Could you check a few things on this model? Use its own coordinates, in mm. Give positions to 0.01 mm unless a question says otherwise; leave off trailing zeros. Order: outer loops, then holes, each group sorted by start corner. A loop starts at its lowest first (then second) coordinate and runs counter-clockwise, first axis right, second up.
(1) Imagine slicing it at A-A, the plane z = 534. Write out the boundary of the cut face in (x, y).
(2) Imagine slicing it at B-B, the plane z = 510. Write out the boundary of the cut face in (x, y), then the cut area to 3 significant figures.
(3) If I drill on probe 1 along X at (y, z) = (39.1, 534); probe 2 along Z at (x, y) = (-13, 35.1); probe 3 along Z at (x, y) = (-14.5, 36.75), over which ranges is the centre line in solid material (lowest first)?
(4) Will these pins go through, and if not, where does the flat tip stop? pin 1 (1.5 mm diameter, centred on y = 37.5, z = 487.5, fed in from -X); pin 2 (3 mm diameter, centred on y = 39.5, z = 473, fed in from +X); pin 3 (3.5 mm diameter, centred on x = 12.39, z = 491.65, fed in from +Y); pin 4 (2.5 mm diameter, centred on x = -7.63, z = 499.9, fed in from -Y).
(5) Imagine slicing it at C-C, the plane y = 39.5. State how many separate pieces and enclosed holes the cut face has, then the cut area to 3 significant figures.
from build123d import *

# Parameters (mm, degrees)
PLACA_START                 = 34.5
SK_PLACA_W                  = 50
SK_PLACA_H                  = 36
PLACA_DEPTH                 = 6
EXTREMO_START               = 34.5
SK_EXTREMO_R                = 25
EXTREMO_DEPTH               = 6
PASANTES_M2_5_CUBO_J5_START = 34.5
SK_PASANTES_M2_5_CUBO_J5_R  = 1.45
PASANTES_M2_5_CUBO_J5_DEPTH = 6
CAJAS_M2_5_J5_START         = 38
SK_CAJAS_M2_5_J5_R          = 2.75
CAJAS_M2_5_J5_DEPTH         = 2.5
EXTENSION_PESTANAS_START    = 34.5
SK_EXTENSION_PESTANAS_W     = 50
SK_EXTENSION_PESTANAS_H     = 19
EXTENSION_PESTANAS_DEPTH    = 6
PASANTES_M4_REPISA_START    = 34.5
SK_PASANTES_M4_REPISA_R     = 2.25
PASANTES_M4_REPISA_DEPTH    = 6
PASANTE_M3_CINCHO_START     = 34.5
SK_PASANTE_M3_CINCHO_R      = 1.7
PASANTE_M3_CINCHO_DEPTH     = 6


with BuildPart() as part:
    # Sk_Placa → Placa (new body)
    with BuildSketch(Plane(origin=(0, 0, 0), x_dir=(1, 0, 0), z_dir=(0, 1, 0)).offset(PLACA_START)):
        with Locations((0, -508)):
            Rectangle(SK_PLACA_W, SK_PLACA_H)
    extrude(amount=PLACA_DEPTH)

    # Sk_Extremo → Extremo (add)
    with BuildSketch(Plane(origin=(0, 0, 0), x_dir=(1, 0, 0), z_dir=(0, 1, 0)).offset(EXTREMO_START)):
        with Locations((0, -490)):
            Circle(SK_EXTREMO_R)
    extrude(amount=EXTREMO_DEPTH)

    # Sk_Pasantes_M2-5_cubo_J5 → Pasantes_M2-5_cubo_J5 (cut)
    with BuildSketch(Plane(origin=(0, 0, 0), x_dir=(1, 0, 0), z_dir=(0, 1, 0)).offset(PASANTES_M2_5_CUBO_J5_START)):
        with Locations(Location((12.390194253, -491.653204878, 0), (0, 0, 270))):
            Circle(SK_PASANTES_M2_5_CUBO_J5_R)
        with Locations(Location((4.763379704, -501.55682542, 0), (0, 0, 270))):
            Circle(SK_PASANTES_M2_5_CUBO_J5_R)
        with Locations(Location((-7.626814549, -499.903620542, 0), (0, 0, 270))):
            Circle(SK_PASANTES_M2_5_CUBO_J5_R)
        with Locations(Location((-12.390194253, -488.346795122, 0), (0, 0, 270))):
            Circle(SK_PASANTES_M2_5_CUBO_J5_R)
        with Locations(Location((-4.763379704, -478.44317458, 0), (0, 0, 270))):
            Circle(SK_PASANTES_M2_5_CUBO_J5_R)
        with Locations(Location((7.626814549, -480.096379458, 0), (0, 0, 270))):
            Circle(SK_PASANTES_M2_5_CUBO_J5_R)
    extrude(amount=PASANTES_M2_5_CUBO_J5_DEPTH, mode=Mode.SUBTRACT)

    # Sk_Cajas_M2-5_J5 → Cajas_M2-5_J5 (cut)
    with BuildSketch(Plane(origin=(0, 0, 0), x_dir=(1, 0, 0), z_dir=(0, 1, 0)).offset(CAJAS_M2_5_J5_START)):
        with Locations(Location((12.390194253, -491.653204878, 0), (0, 0, 270))):
            Circle(SK_CAJAS_M2_5_J5_R)
        with Locations(Location((4.763379704, -501.55682542, 0), (0, 0, 270))):
            Circle(SK_CAJAS_M2_5_J5_R)
        with Locations(Location((-7.626814549, -499.903620542, 0), (0, 0, 270))):
            Circle(SK_CAJAS_M2_5_J5_R)
        with Locations(Location((-12.390194253, -488.346795122, 0), (0, 0, 270))):
            Circle(SK_CAJAS_M2_5_J5_R)
        with Locations(Location((-4.763379704, -478.44317458, 0), (0, 0, 270))):
            Circle(SK_CAJAS_M2_5_J5_R)
        with Locations(Location((7.626814549, -480.096379458, 0), (0, 0, 270))):
            Circle(SK_CAJAS_M2_5_J5_R)
    extrude(amount=CAJAS_M2_5_J5_DEPTH, mode=Mode.SUBTRACT)

    # Sk_Extension_pestanas → Extension_pestanas (add)
    with BuildSketch(Plane(origin=(0, 0, 0), x_dir=(1, 0, 0), z_dir=(0, 1, 0)).offset(EXTENSION_PESTANAS_START)):
        with Locations((0, -535.5)):
            Rectangle(SK_EXTENSION_PESTANAS_W, SK_EXTENSION_PESTANAS_H)
    extrude(amount=EXTENSION_PESTANAS_DEPTH)

    # Sk_Pasantes_M4_repisa → Pasantes_M4_repisa (cut)
    with BuildSketch(Plane(origin=(0, 0, 0), x_dir=(1, 0, 0), z_dir=(0, 1, 0)).offset(PASANTES_M4_REPISA_START)):
        with Locations(Location((-15, -534, 0), (0, 0, 270))):
            Circle(SK_PASANTES_M4_REPISA_R)
        with Locations(Location((15, -534, 0), (0, 0, 270))):
            Circle(SK_PASANTES_M4_REPISA_R)
    extrude(amount=PASANTES_M4_REPISA_DEPTH, mode=Mode.SUBTRACT)

    # Sk_Pasante_M3_cincho → Pasante_M3_cincho (cut)
    with BuildSketch(Plane(origin=(0, 0, 0), x_dir=(1, 0, 0), z_dir=(0, 1, 0)).offset(PASANTE_M3_CINCHO_START)):
        with Locations(Location((-15, -510, 0), (0, 0, 270))):
            Circle(SK_PASANTE_M3_CINCHO_R)
    extrude(amount=PASANTE_M3_CINCHO_DEPTH, mode=Mode.SUBTRACT)


solid = part.part
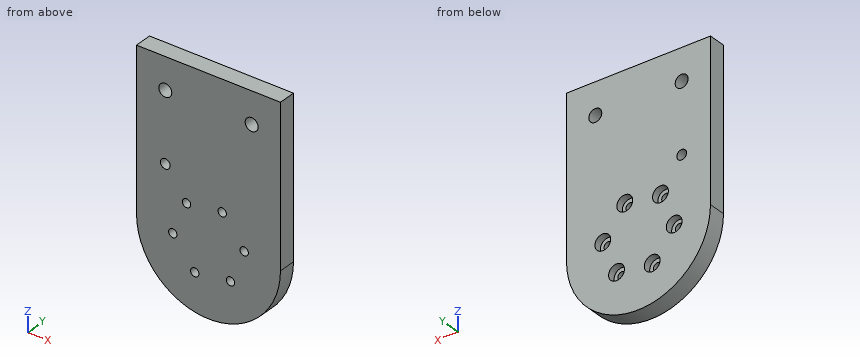
Answer block:
1. outline: (-25, 34.5) - (-17.25, 34.5) - (-17.25, 40.5) - (-25, 40.5) - close; (-12.75, 34.5) - (12.75, 34.5) - (12.75, 40.5) - (-12.75, 40.5) - close; (17.25, 34.5) - (25, 34.5) - (25, 40.5) - (17.25, 40.5) - close
2. outline: (-25, 34.5) - (-16.7, 34.5) - (-16.7, 40.5) - (-25, 40.5) - close; (-13.3, 34.5) - (25, 34.5) - (25, 40.5) - (-13.3, 40.5) - close
2. area: 280 mm2
3. probe 1: x = -25 to -17.25, -12.75 to 12.75, 17.25 to 25
3. probe 2: z = 468.65 to 487.03, 489.66 to 532.97, 535.03 to 545
3. probe 3: z = 469.63 to 508.38, 511.62 to 531.81, 536.19 to 545
4. pin 1: stops at x = -24.94
4. pin 2: stops at x = 19.62
4. pin 3: stops at y = 38
4. pin 4: passes through
5. separate pieces: 1
5. enclosed holes: 9
5. area: 3,550 mm2
